Answer from the drawing. Dimensions are ordinates in mm from the lowest x, y and z of the part. A direction names the side the tool comes from. Give positions to 0.01 mm unless a question says otherwise; leave off trailing zeros. Loops run counter-clockwise (first coordinate to the right, second up) from the corner with the lowest first, then second, coordinate; pieces in that order, holes last. Notation, with made-up numbers: (25, 9.5) -> (53, 9.5) arc R30 cw to (53, 42.5) -> close; hole circle Ø10 at (33, 13). An arc over 180 degrees is marked (long way). Write each question's results on one line, items separated by ' | '. Start each with the question number.
Item 1: Which of the six approach directions +Z, -Z, +X, -X, +Y, -Y give full straight-line access (tool end or side, diameter ignored) to the marked faces 1 and 2?
Item 2: Section B-B on y = 2.75 is taken. Write down the section's boundary in (x, z) (1 decimal), and give its area (3 significant figures).
Item 3: Find the intervals of material crossed by line 1 (X direction, y = 3.75, z = 2.2) (1 decimal); line 2 (Y direction, x = 30.5, z = 1.3), in increasing order.
Item 4: Determine the mould class of the marked faces 3, 4, 5 and 6 for opening direction X: +X half, -X half, draft (parallel to the pull), parting line (faces both ways), or undercut.
Item 5: Section C-C on z = 2.05 is taken. State how many separate pieces and enclosed holes the cut face has, and give its area (3 significant figures).
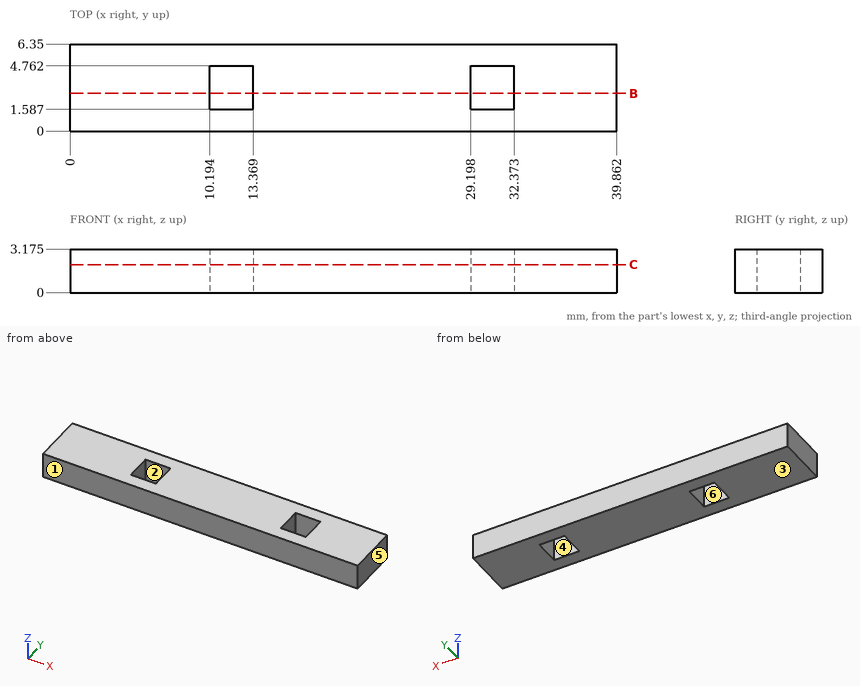
Findings:
1) face 1: +Z, -Z, +X, -X, -Y | face 2: +Z, -Z
2) outline: (0, 0) -> (10.2, 0) -> (10.2, 3.2) -> (0, 3.2) -> close; (13.4, 0) -> (29.2, 0) -> (29.2, 3.2) -> (13.4, 3.2) -> close; (32.4, 0) -> (39.9, 0) -> (39.9, 3.2) -> (32.4, 3.2) -> close | area: 106 mm2
3) line 1: 0 to 10.2, 13.4 to 29.2, 32.4 to 39.9 | line 2: 0 to 1.59, 4.76 to 6.35
4) face 3: draft | face 4: undercut | face 5: +X half | face 6: undercut
5) separate pieces: 1 | enclosed holes: 2 | area: 233 mm2
